The figure shows three views and two pictorial views of one solid part (mm, origin at its lowest corner). Answer the questions. Coordinates: 2 decimals unless noted, no trailing zeros. Write each loop counter-clockwise with the first axis right and the second up, starting at its lowest first coordinate (ties: lowest second). Pieces come first, ordered by that corner, then holes.
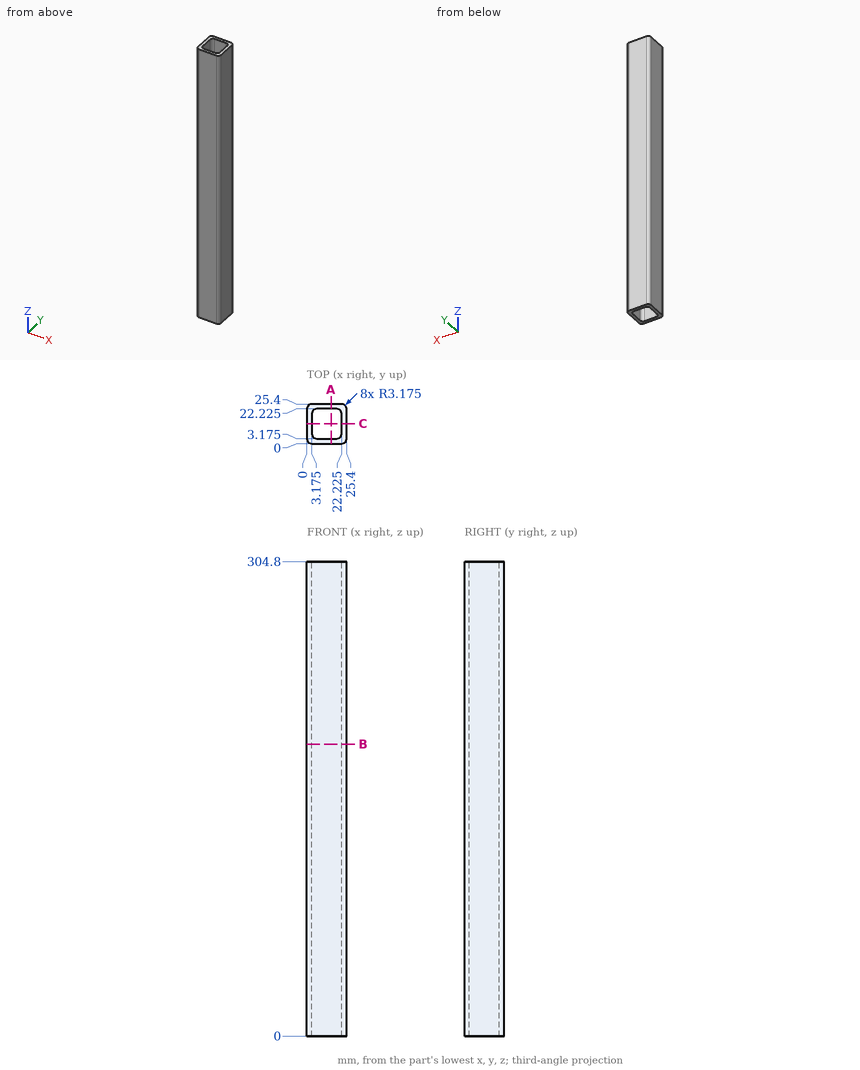
Q1. Find the intervals of material crossed by probe 1 along Y at (x, z) = (15.5, 195) (3 decimals); probe 2 along Y at (x, z) = (3.5, 229), in increasing order.
Answers below:
probe 1: y = 0 to 3.175, 22.225 to 25.4
probe 2: y = 0 to 4.95, 20.45 to 25.4
Q2. The part is cut by section A-A, the plane x = 15.5. Write down the section's boundary in (y, z) (3 decimals).
Answers below:
outline: (0, 0) - (3.175, 0) - (3.175, 304.8) - (0, 304.8) - close; (22.225, 0) - (25.4, 0) - (25.4, 304.8) - (22.225, 304.8) - close
Q3. The part is cut by section B-B, the plane z = 187.5. Write down the section's boundary in (x, y) (3 decimals), then the cut area to 3 significant figures.
Answers below:
outline: (0, 3.175) arc R3.175 ccw to (3.175, 0) - (22.225, 0) arc R3.175 ccw to (25.4, 3.175) - (25.4, 22.225) arc R3.175 ccw to (22.225, 25.4) - (3.175, 25.4) arc R3.175 ccw to (0, 22.225) - close; hole (3.175, 6.35) arc R3.175 ccw to (6.35, 3.175) - (19.05, 3.175) arc R3.175 ccw to (22.225, 6.35) - (22.225, 19.05) arc R3.175 ccw to (19.05, 22.225) - (6.35, 22.225) arc R3.175 ccw to (3.175, 19.05) - close
area: 282 mm2
